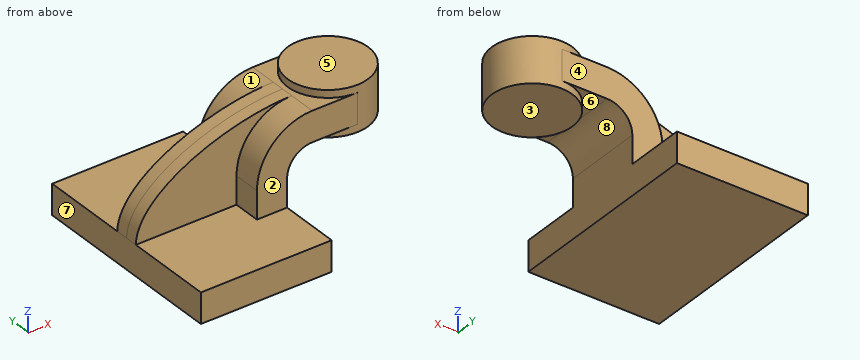
from build123d import *

# Parameters (mm, degrees)
F1_DEPTH = 63.5
F0_W     = 25.4
F0_H     = 19.05
F2_DEPTH = 25.4
F3_DEPTH = 7.9375


with BuildPart() as f1:
    # F0 (on Front) → F1 (new body, symmetric)
    with BuildSketch(Plane.XZ):
        Polygon((-41.275, 9.525), (-41.275, -9.525), (41.275, -9.525), (41.275, 9.525), (22.225, 9.525), align=None)
    extrude(amount=F1_DEPTH, both=True)

    # F0 (on Front) → F2 (join, symmetric)
    with BuildSketch(Plane.XZ):
        with BuildLine():
            Line((60.325, 61.9252), (57.15, 61.9252))
            ThreePointArc((57.15, 61.9252), (32.4542956671, 51.6959043329), (22.225, 27.0002))
            Line((22.225, 27.0002), (22.225, 9.525))
            Line((22.225, 9.525), (41.275, 9.525))
            Line((41.275, 9.525), (41.275, 27.0002))
            ThreePointArc((41.275, 27.0002), (45.9246798487, 38.2255201513), (57.15, 42.8752))
            Line((57.15, 42.8752), (60.325, 42.8752))
            Line((60.325, 42.8752), (60.325, 61.9252))
        make_face()
        with Locations((73.025, 52.4002)):
            Rectangle(F0_W, F0_H)
    extrude(amount=F2_DEPTH, both=True)

    # F0 (on Front) → F3 (join, symmetric)
    with BuildSketch(Plane.XZ):
        with BuildLine():
            add(Edge.make_bspline(
                [(-41.275, 9.525), (-40.5363477767, 39.0089415014), (15.7318022102, 61.9221478701), (57.15, 61.9252)],
                knots=[0, 0, 0, 0, 111.5045361635, 111.5045361635, 111.5045361635, 111.5045361635], degree=3))
            Line((-41.275, 9.525), (22.225, 9.525))
            Line((22.225, 9.525), (22.225, 27.0002))
            ThreePointArc((22.225, 27.0002), (32.4542956671, 51.6959043329), (57.15, 61.9252))
        make_face()
    extrude(amount=F3_DEPTH, both=True)

    # F0 (on Front) → F4 (revolve)
    with BuildSketch(Plane.XZ):
        Polygon((85.725, 66.675), (85.725, 61.9252), (85.725, 42.8752), (85.725, 38.1), (111.125, 38.1), (111.125, 66.675), align=None)
    revolve(axis=Axis((85.725, 0, 52.3875), (0, 0, -1)))


solid = f1.part
CAD build for the part. Positions are in the model's coordinates, mm. Face numbers are marked on the shaded views. A direction names the side the tool comes from. Give positions to 0.01 mm unless a question says otherwise; leave off trailing zeros. Order: outer loops, then holes, each group sorted by start corner. A loop starts at its lowest first (then second) coordinate and runs counter-clockwise, first axis right, second up. Notation, with made-up numbers: (81, 52.25) - (102, 52.25) arc R20 cw to (102, 59.25) - close; hole circle Ø9 at (41.5, -15.5). An arc over 180 degrees is marked (long way). Answer in a Markdown table with one row per item.
1. Saw through at A-A, the plane x = 69. Give the cut face in (y, z) (3 decimals), plus the area to 3 significant figures.
Data:
| item | result |
|---|---|
| outline | (-25.4, 42.875) - (-19.116, 42.875) - (-19.116, 38.1) - (19.116, 38.1) - (19.116, 42.875) - (25.4, 42.875) - (25.4, 61.925) - (19.116, 61.925) - (19.116, 66.675) - (-19.116, 66.675) - (-19.116, 61.925) - (-25.4, 61.925) - close |
| area | 1,330 mm² |
2. Tool access for the marked faces 1, 2, 3 and 4: list every direction of +Z, -Z, +X, -X, +Y, -Y with a clear straight run to the whole face (end or side of a thin tool).
Data:
| item | result |
|---|---|
| face 1 | +Z, -X, +Y |
| face 2 | +Z, +X, -X, -Y |
| face 3 | -Z, +X, +Y, -Y |
| face 4 | +Z, +X, -X, +Y |
3. Pull direction X, two halves, no side cores. Call the marked faces 5, 6, 7 and 8: pulls with the +X half, pulls with the -X half, needs draft (parallel to the pull), parting line crosses it, or undercut.
Data:
| item | result |
|---|---|
| face 5 | needs draft |
| face 6 | undercut |
| face 7 | pulls with the -X half |
| face 8 | undercut |
4. Saw through at D-D, the plane x = 97.5. Give the cut face in (y, z) (3 decimals), plus the area to 3 significant figures.
Data:
| item | result |
|---|---|
| outline | (-22.506, 38.1) - (22.506, 38.1) - (22.506, 66.675) - (-22.506, 66.675) - close |
| area | 1,290 mm² |
5. Saw through at B-B, the plane y = 23.5. Give the cut face in (x, z) (3 decimals).
Data:
| item | result |
|---|---|
| outline | (-41.275, -9.525) - (41.275, -9.525) - (41.275, 27) arc R15.875 cw to (57.15, 42.875) - (76.086, 42.875) - (76.086, 38.1) - (95.364, 38.1) - (95.364, 66.675) - (76.086, 66.675) - (76.086, 61.925) - (57.15, 61.925) arc R34.925 ccw to (22.225, 27) - (22.225, 9.525) - (-41.275, 9.525) - close |
6. Saw through at C-C, the plane y = -47. Give the cut face in (x, z) (3 decimals).
Data:
| item | result |
|---|---|
| outline | (-41.275, -9.525) - (41.275, -9.525) - (41.275, 9.525) - (-41.275, 9.525) - close |
7. Flat gauge pins, fed straight in: pin 1 (2 mm diameter, centred on x = 37.5, z = 52, fed in from +Y); pin 2 (14 mm diameter, centred on y = -13, z = 18, fed in from -X); pin 3 (5 mm diameter, centred on y = 20.5, z = 18.5, fed in from -X) (3 decimals). Where does each tip first touch, or does it go through?
Data:
| item | result |
|---|---|
| pin 1 | stops at y = 25.4 |
| pin 2 | stops at x = -40.9 |
| pin 3 | stops at x = 22.225 |
8. Probe probe 1 along Z at (x, y) = (1.5, -50) (3 decimals); probe 2 along Z at (x, y) = (98, 6) (3 decimals); probe 3 along X at (y, z) = (23, 24.5) (3 decimals). List the from-to ranges inside material, lowest first. Write a range as [from, to].
Data:
| item | result |
|---|---|
| probe 1 | z = [-9.525, 9.525] |
| probe 2 | z = [38.1, 66.675] |
| probe 3 | x = [22.225, 41.275] |
